Source: three-view drawing plus pictorial views. Frame: mm from the lowest corner of the part. A direction names the side the tool comes from. Coordinates: 2 decimals unless noted, no trailing zeros. Order: outer loops, then holes, each group sorted by start corner. A loop starts at its lowest first (then second) coordinate and runs counter-clockwise, first axis right, second up. Notation, with made-up numbers: (53, 8.25) - (96, 8.25) arc R27 ccw to (96, 31.25) - close; hole circle Ø5 at (41.5, 5.25). An arc over 180 degrees is marked (long way). One line per question, with ' | ' between items.
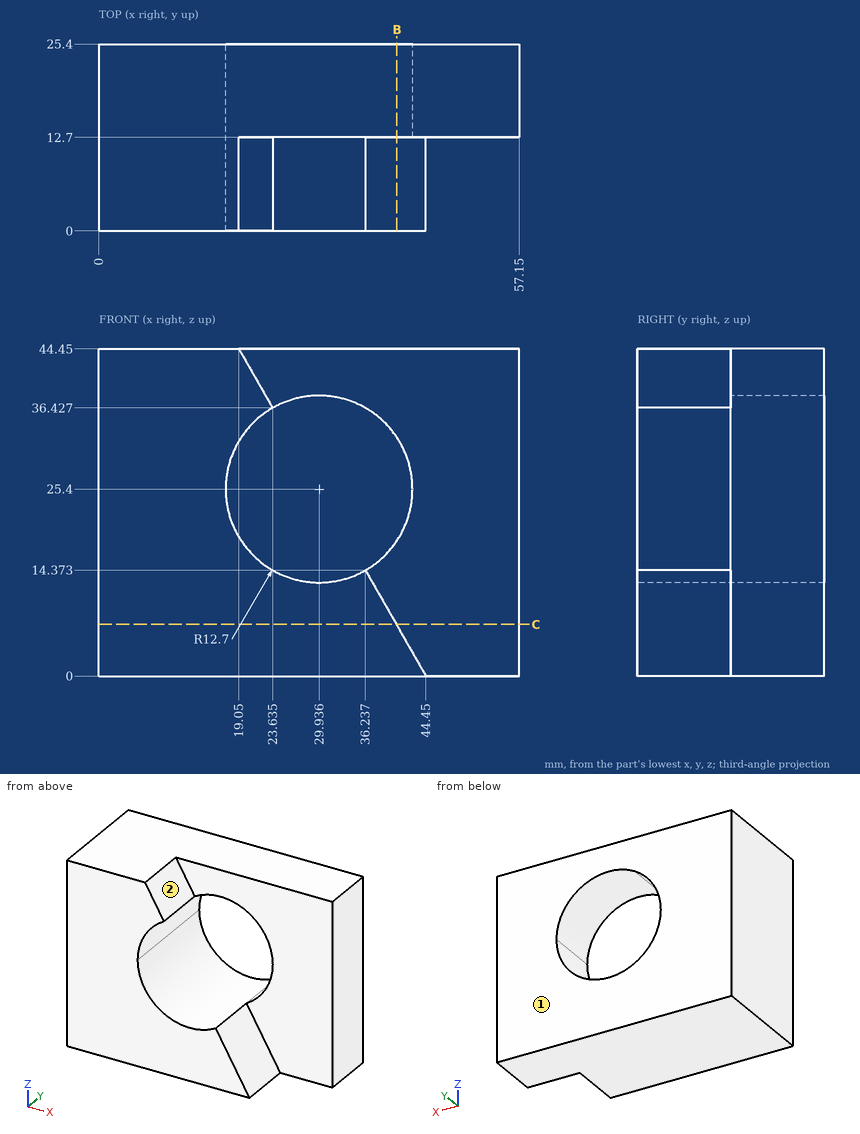
(1) Cut plane B-B (x = 40.5). Return the cut outline in (y, z).
Taken from the geometry:
outline: (0, 0) - (25.4, 0) - (25.4, 18.35) - (12.7, 18.35) - (12.7, 6.91) - (0, 6.91) - close; (12.7, 32.45) - (25.4, 32.45) - (25.4, 44.45) - (12.7, 44.45) - close
(2) Material intervals for L1, parallel to X at y = 16.75, z = 26; L2, parallel to Y at x = 50, z = 38; L3, parallel to Z at x = 19.5, y = 3.25 (1 decimal), sorted ascending. Write a range as from..to.
Taken from the geometry:
L1: x = 0..17.25, 42.62..57.15 | L2: y = 12.7..25.4 | L3: z = 0..18.2, 32.6..43.7
(3) Set-up query: the marked faces 1 and 2. Return all of +Z, -Z, +X, -X, +Y, -Y with unobstructed straight access to the full face (end or side cutting, diameter ignored); none if empty.
Taken from the geometry:
face 1: +Z, -Z, +X, -X, +Y | face 2: +Z, +X, -Y
(4) Cut plane C-C (z = 7). Return the cut outline in (x, y), and give its area (3 significant figures).
Taken from the geometry:
outline: (0, 0) - (40.45, 0) - (40.45, 12.7) - (57.15, 12.7) - (57.15, 25.4) - (0, 25.4) - close | area: 1,240 mm²
(5) Pin query (flat end, axial travel): P1, Ø4, axis at x = 19.5, y = 7, coming from the +Z side; P2, Ø3, axis at x = 47, z = 22.5, coming from the -Y side; P3, Ø3, axis at y = 6, z = 37, coming from the +X side (1 decimal); P4, Ø12, axis at y = 6, z = 27.5, coming from the +X side (1 decimal). Return the tip coordinate at first contact, or that it passes through.
Taken from the geometry:
P1: stops at z = 44.45 | P2: stops at y = 12.7 | P3: stops at x = 23.6 | P4: stops at x = 20.2
